Read the model definition and answer for the solid it produces. Units are mm, in the model's axes. Face numbers are marked on the shaded views. Give positions to 0.01 mm unless a question says otherwise; leave off trailing zeros. Order: outer loops, then holes, each group sorted by start corner. A loop starts at its lowest first (then second) coordinate and runs counter-clockwise, first axis right, second up. Notation, with made-up numbers: (25.5, 31) - (36.5, 31) arc R35 ccw to (36.5, 66) - close; hole circle Ø9 at (24, 80.5). An arc over 180 degrees is marked (long way). Write each question's results on one line, items separated by ' | '. Start each with the question number.
Q1. For a pull along Z with two mould halves and no side action, classify the marked faces 1 and 2 as +Z half, -Z half, draft (parallel to the pull), parting line (faces both ways), or undercut.
Q2. Find section B-B on y = 3.3. Give the vertices of the cut face in (x, z).
Q3. Find the intervals of material crossed by line 1 along X through (y, z) = (1.9, 7.5); line 2 along X through (y, z) = (1.2, 0); line 3 along Z through (x, y) = (46, 1.4), in increasing order. Write a range as from..to.
Q4. Find section C-C on z = -40. Give the vertices of the cut face in (x, y), and give its area (3 significant figures).
Q5. Flat-ended cylindrical pins translate along their axes: P1, Ø1.8, axis at x = 23, z = -40, coming from the +Y side; P2, Ø10, axis at x = 5.5, z = -28.5, coming from the +Y side; P3, Ø0.6, axis at x = 25.5, y = 1, coming from the +Z side. Find the tip coordinate at first contact, or state that the pin passes through.
Q6. Find section A-A on z = 0. Give the vertices of the cut face in (x, y), and give its area (3 significant figures).
Q7. Find section D-D on z = -21.5. Give the vertices of the cut face in (x, y).
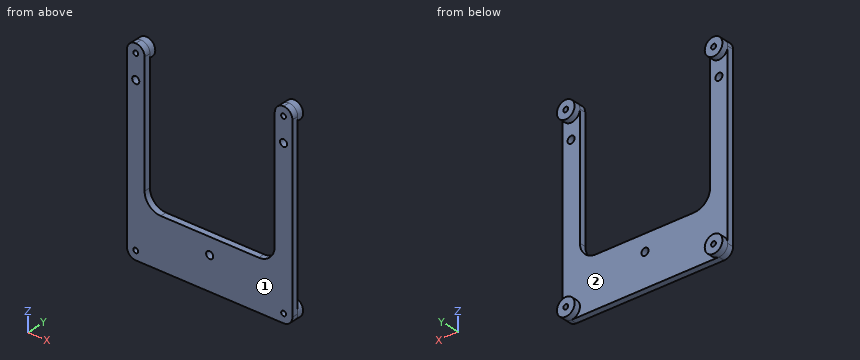
from build123d import *

# Parameters (mm, degrees)
SKETCH2_W               = 54
SKETCH2_H               = 63
SKETCH2_R               = 0.75
BOSS_EXTRUDE1_DEPTH     = 2
SKETCH1_R               = 1.1
CUT_EXTRUDE2_DEPTH      = 3
CUT_EXTRUDE2_DEPTH_BACK = 1
SKETCH3_R               = 2.75
SKETCH3_R_2             = 0.75
BOSS_EXTRUDE2_DEPTH     = 2
SKETCH4_OUTSIDE_W       = 72.614
SKETCH4_OUTSIDE_H       = 81.614
CUT_EXTRUDE3_DEPTH      = 3
CUT_EXTRUDE3_DEPTH_BACK = 3
CUT_EXTRUDE4_DEPTH      = 3
CUT_EXTRUDE4_DEPTH_BACK = 3
FILLET1_R               = 5


with BuildPart() as part:
    # Sketch2 → Boss-Extrude1 (new body)
    with BuildSketch(Plane(origin=(0, 0, 0), x_dir=(1, 0, 0), z_dir=(0, 1, 0))):
        with Locations((23, 20)):
            Rectangle(SKETCH2_W, SKETCH2_H)
        with Locations((46, -7.5)):
            Circle(SKETCH2_R, mode=Mode.SUBTRACT)
        with Locations((46, 47.5)):
            Circle(SKETCH2_R, mode=Mode.SUBTRACT)
        with Locations((0, 47.5)):
            Circle(SKETCH2_R, mode=Mode.SUBTRACT)
        with Locations((0, -7.5)):
            Circle(SKETCH2_R, mode=Mode.SUBTRACT)
    extrude(amount=BOSS_EXTRUDE1_DEPTH)

    # Sketch1 → Cut-Extrude2 (cut, two sides)
    with BuildSketch(Plane(origin=(0, 0, 0), x_dir=(1, 0, 0), z_dir=(0, 1, 0))) as cut_extrude2_sk:
        Circle(SKETCH1_R)
        with Locations((46, 0)):
            Circle(SKETCH1_R)
        with Locations((23, 40)):
            Circle(SKETCH1_R)
    extrude(amount=CUT_EXTRUDE2_DEPTH, mode=Mode.SUBTRACT)
    extrude(cut_extrude2_sk.sketch, amount=-CUT_EXTRUDE2_DEPTH_BACK, mode=Mode.SUBTRACT)

    # Sketch3 → Boss-Extrude2 (add)
    with BuildSketch(Plane(origin=(0, 2, 0), x_dir=(1, 0, 0), z_dir=(0, 1, 0))):
        with Locations((0, -7.5)):
            Circle(SKETCH3_R)
        with Locations((0, -7.5)):
            Circle(SKETCH3_R_2, mode=Mode.SUBTRACT)
        with Locations((46, -7.5)):
            Circle(SKETCH3_R)
        with Locations((46, -7.5)):
            Circle(SKETCH3_R_2, mode=Mode.SUBTRACT)
        with Locations((46, 47.5)):
            Circle(SKETCH3_R)
        with Locations((46, 47.5)):
            Circle(SKETCH3_R_2, mode=Mode.SUBTRACT)
        with Locations((0, 47.5)):
            Circle(SKETCH3_R)
        with Locations((0, 47.5)):
            Circle(SKETCH3_R_2, mode=Mode.SUBTRACT)
    extrude(amount=BOSS_EXTRUDE2_DEPTH)

    # Sketch4 outside → Cut-Extrude3 (cut, two sides)
    with BuildSketch(Plane(origin=(0, 2, 0), x_dir=(1, 0, 0), z_dir=(0, 1, 0))) as cut_extrude3_sk:
        with Locations((23, 20)):
            Rectangle(SKETCH4_OUTSIDE_W, SKETCH4_OUTSIDE_H)
        with BuildLine():
            Line((0, -10.25), (46, -10.25))
            ThreePointArc((46, -10.25), (47.944543648, -9.444543648), (48.75, -7.5))
            Line((48.75, -7.5), (48.75, 47.5))
            ThreePointArc((48.75, 47.5), (47.944543648, 49.444543648), (46, 50.25))
            Line((46, 50.25), (0, 50.25))
            ThreePointArc((0, 50.25), (-1.944543648, 49.444543648), (-2.75, 47.5))
            Line((-2.75, 47.5), (-2.75, -7.5))
            ThreePointArc((-2.75, -7.5), (-1.944543648, -9.444543648), (0, -10.25))
        make_face(mode=Mode.SUBTRACT)
    extrude(amount=CUT_EXTRUDE3_DEPTH, mode=Mode.SUBTRACT)
    extrude(cut_extrude3_sk.sketch, amount=-CUT_EXTRUDE3_DEPTH_BACK, mode=Mode.SUBTRACT)

    # Sketch5 → Cut-Extrude4 (cut, two sides)
    with BuildSketch(Plane(origin=(0, 2, 0), x_dir=(1, 0, 0), z_dir=(0, 1, 0))) as cut_extrude4_sk:
        with BuildLine():
            Line((2.75, 34.9), (2.75, -7.5))
            ThreePointArc((2.75, -7.5), (1.944543648, -9.444543648), (0, -10.25))
            Line((0, -10.25), (46, -10.25))
            ThreePointArc((46, -10.25), (44.055456352, -9.444543648), (43.25, -7.5))
            Line((43.25, -7.5), (43.25, 34.9))
            Line((43.25, 34.9), (2.75, 34.9))
        make_face()
    extrude(amount=CUT_EXTRUDE4_DEPTH, mode=Mode.SUBTRACT)
    extrude(cut_extrude4_sk.sketch, amount=-CUT_EXTRUDE4_DEPTH_BACK, mode=Mode.SUBTRACT)

    # Fillet1
    fillet1_edges = [part.edges().sort_by_distance(p)[0] for p in [
        (2.75, 1, -34.9),
        (43.25, 1, -34.9),
    ]]
    fillet(fillet1_edges, radius=FILLET1_R)


solid = part.part
Working result:
1) face 1: draft | face 2: undercut
2) outline: circle Ø5.5 at (0, -47.5); circle Ø5.5 at (0, 7.5); circle Ø5.5 at (46, -47.5); circle Ø5.5 at (46, 7.5); hole circle Ø1.5 at (0, -47.5); hole circle Ø1.5 at (0, 7.5); hole circle Ø1.5 at (46, -47.5); hole circle Ø1.5 at (46, 7.5)
3) line 1: -2.75..-0.75, 0.75..2.75, 43.25..45.25, 46.75..48.75 | line 2: -2.75..-1.1, 1.1..2.75, 43.25..44.9, 47.1..48.75 | line 3: -50.25..-48.25, -46.75..-1.1, 1.1..6.75, 8.25..10.25
4) outline: (-2.75, 0) - (21.9, 0) - (21.9, 2) - (-2.75, 2) - close; (24.1, 0) - (48.75, 0) - (48.75, 2) - (24.1, 2) - close | area: 98.6 mm²
5) P1: through | P2: y = 2 | P3: z = -34.9
6) outline: (-2.75, 0) - (-1.1, 0) - (-1.1, 2) - (-2.75, 2) - close; (1.1, 0) - (2.75, 0) - (2.75, 2) - (1.1, 2) - close; (43.25, 0) - (44.9, 0) - (44.9, 2) - (43.25, 2) - close; (47.1, 0) - (48.75, 0) - (48.75, 2) - (47.1, 2) - close | area: 13.2 mm²
7) outline: (-2.75, 0) - (2.75, 0) - (2.75, 2) - (-2.75, 2) - close; (43.25, 0) - (48.75, 0) - (48.75, 2) - (43.25, 2) - close
